Geometry check sheet. Reference: the model listing, model coordinates, mm. Face numbers are marked on the shaded views. A direction names the side the tool comes from. Coordinates: 2 decimals unless noted, no trailing zeros. Write each loop counter-clockwise with the first axis right and the second up, starting at its lowest first coordinate (ties: lowest second). Pieces come first, ordered by that corner, then holes. Notation, with made-up numbers: M 20,74 L 32,74 A19 cw 32,109 Z; hole C -4.75,-19 d9. An arc over 180 degrees is marked long. Write each question's results on one line, items separated by ' | '.
```python
from build123d import *

# Parameters (mm, degrees)
SKETCH1_W               = 7
SKETCH1_H               = 5.5
BOSS_EXTRUDE1_DEPTH     = 6.5
SKETCH4_W               = 5.5
SKETCH4_H               = 3
CUT_EXTRUDE1_DEPTH      = 10.20597632
BOSS_EXTRUDE2_DEPTH     = 1
BOSS_EXTRUDE3_DEPTH     = 1
SKETCH8_R               = 2.25
CUT_EXTRUDE2_DEPTH      = 2
BOSS_EXTRUDE4_DEPTH     = 3.6
SKETCH11_R              = 1
BOSS_EXTRUDE5_DEPTH     = 7.5
FILLET1_R               = 0.5
SKETCH12_W              = 0.75
SKETCH12_H              = 3
BOSS_EXTRUDE6_DEPTH     = 1
SKETCH14_W              = 0.75
SKETCH14_H              = 1
BOSS_EXTRUDE7_DEPTH     = 0.5
CUT_EXTRUDE3_DEPTH      = 14.419109508
CUT_EXTRUDE3_DEPTH_BACK = 14.419109508


with BuildPart() as part:
    # Sketch1 → Boss-Extrude1 (new body)
    with BuildSketch(Plane(origin=(0, 0, 0), x_dir=(1, 0, 0), z_dir=(0, 1, 0))):
        Rectangle(SKETCH1_W, SKETCH1_H)
    extrude(amount=BOSS_EXTRUDE1_DEPTH)

    # Sketch4 → Cut-Extrude1 (cut, through all)
    with BuildSketch(Plane.XY.offset(2.75)):
        with Locations((0, 1.5)):
            Rectangle(SKETCH4_W, SKETCH4_H)
    extrude(amount=-CUT_EXTRUDE1_DEPTH, mode=Mode.SUBTRACT)

    # Sketch6 → Boss-Extrude2 (add)
    with BuildSketch(Plane.ZY.offset(3.5)):
        Polygon((-1, 4.5), (-0.75, 4.5), (-0.75, 5), (0.75, 5), (0.75, 4.5), (1, 4.5), (1, 0), (-1, 0), align=None)
    extrude(amount=BOSS_EXTRUDE2_DEPTH)

    # Sketch7 → Boss-Extrude3 (add)
    with BuildSketch(Plane(origin=(3.5, 0, 0), x_dir=(0, 0, -1), z_dir=(1, 0, 0))):
        Polygon((-1, 0), (-1, 4.5), (-0.75, 4.5), (-0.75, 5), (0.75, 5), (0.75, 4.5), (1, 4.5), (1, 0), align=None)
    extrude(amount=BOSS_EXTRUDE3_DEPTH)

    # Sketch8 → Cut-Extrude2 (cut)
    with BuildSketch(Plane.XZ.offset(-3)):
        with Locations(Location((0, 0, 0), (0, 0, 270))):
            Circle(SKETCH8_R)
    extrude(amount=-CUT_EXTRUDE2_DEPTH, mode=Mode.SUBTRACT)

    # Sketch10 → Boss-Extrude4 (add)
    with BuildSketch(Plane(origin=(0, 6.5, 0), x_dir=(1, 0, 0), z_dir=(0, 1, 0))):
        Polygon((-2.05, -0.675), (-2.05, 0.675), (-0.675, 0.675), (-0.675, 2.05), (0.675, 2.05), (0.675, 0.675), (2.05, 0.675), (2.05, -0.675), (0.675, -0.675), (0.675, -2.05), (-0.675, -2.05), (-0.675, -0.675), align=None)
    extrude(amount=BOSS_EXTRUDE4_DEPTH)

    # Sketch11 → Boss-Extrude5 (add)
    with BuildSketch(Plane.XZ.offset(-5)):
        with Locations(Location((0, 0, 0), (0, 0, 270))):
            Circle(SKETCH11_R)
    extrude(amount=BOSS_EXTRUDE5_DEPTH)

    # Fillet1
    fillet1_edges = [part.edges().sort_by_distance(p)[0] for p in [
        (0, -2.5, 1),
    ]]
    fillet(fillet1_edges, radius=FILLET1_R)

    # Sketch12 → Boss-Extrude6 (add)
    with BuildSketch(Plane(origin=(0, 0, -2.75), x_dir=(-1, 0, 0), z_dir=(0, 0, -1))):
        with Locations((-3.125, 1.5)):
            Rectangle(SKETCH12_W, SKETCH12_H)
        with Locations((3.125, 1.5)):
            Rectangle(SKETCH12_W, SKETCH12_H)
    extrude(amount=BOSS_EXTRUDE6_DEPTH)

    # Sketch14 → Boss-Extrude7 (add)
    with BuildSketch(Plane.XZ):
        with Locations((-3.125, -3.25)):
            Rectangle(SKETCH14_W, SKETCH14_H)
        with Locations((3.125, -3.25)):
            Rectangle(SKETCH14_W, SKETCH14_H)
    extrude(amount=BOSS_EXTRUDE7_DEPTH)

    # Sketch15 → Cut-Extrude3 (cut, two sides: drawn at the far end of the back side and taken through both)
    with BuildSketch(Plane(origin=(3.5, 0, 0), x_dir=(0, 0, -1), z_dir=(1, 0, 0)).offset(-CUT_EXTRUDE3_DEPTH_BACK)):
        Polygon((3.75, 3), (3.25, 3), (3.75, -0.5), align=None)
        Polygon((2.75, 0), (3.05, 0), (3.121428571, -0.5), (2.75, -0.5), align=None)
    extrude(amount=CUT_EXTRUDE3_DEPTH + CUT_EXTRUDE3_DEPTH_BACK, mode=Mode.SUBTRACT)


solid = part.part
```
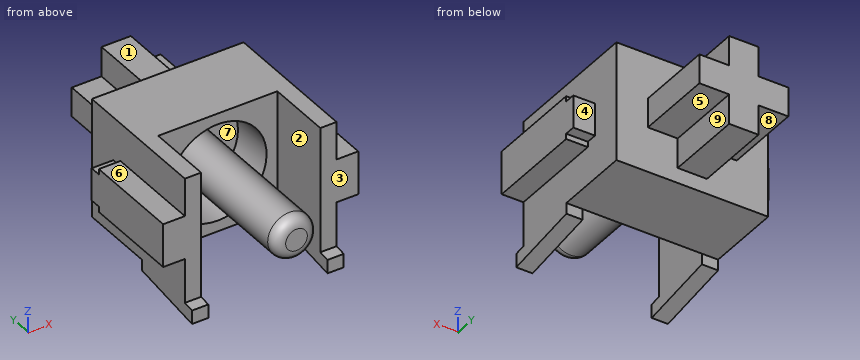
Q1. Mould release check, pull along Z, two halves, no side actions. Record for the marked faces 6, 7, 8 and 9: pulls with the +Z half, pulls with the -Z half, needs draft (parallel to the pull), parting line crosses it, or undercut.
Geometry check:
face 6: pulls with the +Z half | face 7: undercut | face 8: pulls with the -Z half | face 9: needs draft
Q2. Sectioned sample at B-B on x = 3. Record the cut outline in (y, z).
Geometry check:
outline: M -0.5,-3.75 L 3,-3.25 L 3,-2.75 L 6.5,-2.75 L 6.5,2.75 L 0,2.75 L 0,-3.05 L -0.5,-3.12 Z
Q3. Sectioned sample at A-A on y = 4.75. Record the cut outline in (x, z).
Geometry check:
outline: M -4.5,-0.75 L -3.5,-0.75 L -3.5,-2.75 L 3.5,-2.75 L 3.5,-0.75 L 4.5,-0.75 L 4.5,0.75 L 3.5,0.75 L 3.5,2.75 L -3.5,2.75 L -3.5,0.75 L -4.5,0.75 Z; C 0,0 d2; hole C 0,0 d4.5
Q4. Depth check by flat-ended pin: P1, Ø1.5, axis at y = 8.5, z = -1.5, coming from the +X side (3 decimals); P2, Ø3, axis at y = 5.5, z = -0.5, coming from the +X side; P3, Ø0.7, axis at x = 1.5, y = 8, coming from the +Z side (3 decimals); P4, Ø0.8, axis at x = 4, y = 3, coming from the +Z side. Enter the tip coordinate at first touch or a pass-through.
Geometry check:
P1: stops at x = 0.675 | P2: stops at x = 4.5 | P3: stops at z = 0.675 | P4: stops at z = 1
Q5. Access from +Z, -Z, +X, -X, +Y, -Y to the whole of each face (thin tool, end or side, straight path). Record for the marked faces 1, 2, 3, 4 and 5.
Geometry check:
face 1: +Z, +X, -X, +Y | face 2: +Z, -Z, -Y | face 3: +Z, +X, -Y | face 4: +Z, -Z, +X, +Y | face 5: -Z, +X, +Y
Q6. Scan lines: probe 1 along X at (y, z) = (4.65, 0); probe 2 along Y at (x, z) = (-1.25, 2); probe 3 along X at (y, z) = (3.75, -0.5). Record each from-to range of solid material in increasing order.
Geometry check:
probe 1: x = -4.5 to -2.25, -1 to 1, 2.25 to 4.5 | probe 2: y = 3 to 6.5 | probe 3: x = -4.5 to -2.19, -0.87 to 0.87, 2.19 to 4.5
Q7. Sectioned sample at C-C on y = 9. Record the cut outline in (x, z) (3 decimals).
Geometry check:
outline: M -2.05,-0.675 L -0.675,-0.675 L -0.675,-2.05 L 0.675,-2.05 L 0.675,-0.675 L 2.05,-0.675 L 2.05,0.675 L 0.675,0.675 L 0.675,2.05 L -0.675,2.05 L -0.675,0.675 L -2.05,0.675 Z
